Source: CAD feature listing. Evaluate the final solid. Frame: model axes, mm. A direction names the side the tool comes from. Give positions to 0.01 mm unless a question says otherwise; leave off trailing zeros. Order: outer loops, then holes, each group sorted by start corner. A loop starts at its lowest first (then second) coordinate and runs counter-clockwise, first axis right, second up.
from build123d import *

# Parameters (mm, degrees)
F2_DEPTH = 17.78
F1_R     = 4.1275
F3_DEPTH = 1.7145


with BuildPart() as f2:
    # F1 (on Top) → F2 (new body)
    with BuildSketch(Plane.XY):
        Polygon((-271.632484, 50.297177), (-247.819984, 9.052717), (-271.632484, -32.191743), (-247.819984, -73.436203), (-200.194984, -73.436203), (-176.382484, -114.680663), (-128.757484, -114.680663), (-104.944984, -155.925123), (-57.319984, -155.925123), (-33.507484, -114.680663), (14.117516, -114.680663), (37.930016, -73.436203), (85.555016, -73.436203), (109.367516, -32.191743), (85.555016, 9.052717), (109.367516, 50.297177), (85.555016, 91.541636), (109.367516, 132.786096), (85.555016, 174.030556), (37.930016, 174.030556), (14.117516, 215.275016), (-33.507484, 215.275016), (-57.319984, 256.519476), (-104.944984, 256.519476), (-128.757484, 215.275016), (-176.382484, 215.275016), (-200.194984, 174.030556), (-247.819984, 174.030556), (-271.632484, 132.786096), (-247.819984, 91.541636), align=None)
        with BuildLine():
            ThreePointArc((-109.707484, 72.522177), (-107.847612, 77.012305), (-103.357484, 78.872177))
            Line((-103.357484, 78.872177), (-58.907484, 78.872177))
            ThreePointArc((-58.907484, 78.872177), (-54.417356, 77.012305), (-52.557484, 72.522177))
            Line((-52.557484, 72.522177), (-52.557484, 28.072177))
            ThreePointArc((-52.557484, 28.072177), (-54.417356, 23.582049), (-58.907484, 21.722177))
            Line((-58.907484, 21.722177), (-103.357484, 21.722177))
            ThreePointArc((-103.357484, 21.722177), (-107.847612, 23.582049), (-109.707484, 28.072177))
            Line((-109.707484, 28.072177), (-109.707484, 72.522177))
        make_face(mode=Mode.SUBTRACT)
    extrude(amount=F2_DEPTH)

    # F1 (on Top) → F3 (join)
    with BuildSketch(Plane.XY):
        with BuildLine():
            Line((-58.907484, 78.872177), (-103.357484, 78.872177))
            ThreePointArc((-103.357484, 78.872177), (-107.847612, 77.012305), (-109.707484, 72.522177))
            Line((-109.707484, 72.522177), (-109.707484, 28.072177))
            ThreePointArc((-109.707484, 28.072177), (-107.847612, 23.582049), (-103.357484, 21.722177))
            Line((-103.357484, 21.722177), (-58.907484, 21.722177))
            ThreePointArc((-58.907484, 21.722177), (-54.417356, 23.582049), (-52.557484, 28.072177))
            Line((-52.557484, 28.072177), (-52.557484, 72.522177))
            ThreePointArc((-52.557484, 72.522177), (-54.417356, 77.012305), (-58.907484, 78.872177))
        make_face()
        with Locations((-81.132484, 50.297177)):
            Circle(F1_R, mode=Mode.SUBTRACT)
    extrude(amount=F3_DEPTH)


solid = f2.part
(1) Pin query (flat end, axial travel): pin 1 Ø2 at (y, z) = (12.5, 2.5) entering from -X; pin 2 Ø10 at (y, z) = (151.5, 10.5) entering from -X; pin 3 Ø9 at (x, z) = (-144.5, 8.5) entering from +Y (3 decimals). Return the tip coordinate at first contact, or that it passes through.
(2) Section C-C, the plane x = -11. Return loops of the section in (y, z).
(3) Section A-A, the plane x = -90.5. Return loops of the section in (y, z).
(4) Access query for faces 1 (the flat face through (-152, 215.275, 9)), 2 (the flat face through (-81, 21.722, 10)), 3 (the flat face through (-259.89, 112.45, 8.77)). Directions: +Z, -Z, +X, -X, +Y, -Y. A direction counts if a zero-diameter tool reaches every point of the face in a straight line with its end or side. Return the directions, or none.
(5) Line query: line 1 along Y through (x, z) = (-248.5, 11); line 2 along Y through (x, z) = (-80, 13); line 3 along Y through (x, z) = (-256, 5.5). Output: solid intervals per line, ascending.
(6) Section B-B, the plane y = -67. Return loops of the section in (x, z).
(7) Draft query along Y for faces 4 (the flat face through (-41, 53, 0)), 5 (the flat face through (97.295, 29.386, 8.766)), 6 (the flat face through (-116.68, 236.19, 8.77)), 7 (the flat face through (-153, -114.681, 9)). Return one class per face: +Y half, -Y half, draft (parallel to the pull), parting line (faces both ways), or undercut.
Checks:
1. pin 1: stops at x = -250.39
1. pin 2: stops at x = -263.71
1. pin 3: stops at y = 215.275
2. outline: (-114.68, 0) - (215.28, 0) - (215.28, 17.78) - (-114.68, 17.78) - close
3. outline: (-155.93, 0) - (256.52, 0) - (256.52, 17.78) - (78.87, 17.78) - (78.87, 1.71) - (21.72, 1.71) - (21.72, 17.78) - (-155.93, 17.78) - close
4. face 1: +Z, -Z, -X, +Y
4. face 2: +Z
4. face 3: +Z, -Z, -X
5. line 1: y = -72.26 to 7.87, 10.23 to 90.36, 92.72 to 172.85
5. line 2: y = -155.93 to 21.72, 78.87 to 256.52
5. line 3: y = -59.27 to -5.12, 23.22 to 77.37, 105.71 to 159.86
6. outline: (-251.54, 0) - (89.27, 0) - (89.27, 17.78) - (-251.54, 17.78) - close
7. face 4: draft
7. face 5: undercut
7. face 6: +Y half
7. face 7: -Y half
